from build123d import *

# Parameters (mm, degrees)
SKETCH_1_R          = 3
EXTRUDE_1_DEPTH     = 12
CUT_EXTRUDE_1_DEPTH = 41.249223595
CUT_EXTRUDE_2_DEPTH = 23
SKETCH_4_R          = 2
CUT_EXTRUDE_3_DEPTH = 3
SKETCH_4_2_R        = 2
CUT_EXTRUDE_4_DEPTH = 41.249223625


with BuildPart() as part:
    # Sketch 1 → Extrude 1 (new body)
    with BuildSketch(Plane(origin=(0, 0, 0), x_dir=(1, 0, 0), z_dir=(0, 1, 0))):
        with BuildLine():
            Line((0, 0), (30, 0))
            Line((30, 0), (30, -24))
            Line((30, -24), (10.696938457, -24))
            ThreePointArc((10.696938457, -24), (8.799571861, -23.323790008), (7.757550765, -21.6))
            ThreePointArc((7.757550765, -21.6), (5.601317771, -16.801757364), (1.6, -13.386800671))
            ThreePointArc((1.6, -13.386800671), (0.430953484, -12.282694177), (0, -10.733500839))
            Line((0, -10.733500839), (0, 0))
        make_face()
        with Locations(Location((12, -20, 0), (0, 0, 270))):
            Circle(SKETCH_1_R, mode=Mode.SUBTRACT)
        with Locations(Location((25, -20, 0), (0, 0, 270))):
            Circle(SKETCH_1_R, mode=Mode.SUBTRACT)
    extrude(amount=EXTRUDE_1_DEPTH)

    # Sketch 2 → Cut-Extrude 1 (cut, through all)
    with BuildSketch(Plane(origin=(0, 0, 0), x_dir=(-1, 0, 0), z_dir=(0, 0, -1))):
        with BuildLine():
            Line((-30, 12), (-30, 0))
            ThreePointArc((-30, 0), (-28.649110641, 6), (-30, 12))
        make_face()
    extrude(amount=-CUT_EXTRUDE_1_DEPTH, mode=Mode.SUBTRACT)

    # Sketch 3 → Cut-Extrude 2 (cut)
    with BuildSketch(Plane.ZY):
        Polygon((0, 2.75), (0, 9.25), (4.253461365, 10), (4.253461365, 2), align=None)
    extrude(amount=-CUT_EXTRUDE_2_DEPTH, mode=Mode.SUBTRACT)

    # Sketch 4 → Cut-Extrude 3 (cut)
    with BuildSketch(Plane.ZY):
        with BuildLine():
            Line((4.253461365, 10), (4.253461365, 2))
            ThreePointArc((4.253461365, 2), (11.421253901, 6), (4.253461365, 10))
        make_face()
        with Locations((6.721253901, 6)):
            Circle(SKETCH_4_R, mode=Mode.SUBTRACT)
    extrude(amount=-CUT_EXTRUDE_3_DEPTH, mode=Mode.SUBTRACT)

    # Sketch 4_2 → Cut-Extrude 4 (cut, through all)
    with BuildSketch(Plane.ZY):
        with Locations((6.721253901, 6)):
            Circle(SKETCH_4_2_R)
    extrude(amount=-CUT_EXTRUDE_4_DEPTH, mode=Mode.SUBTRACT)


solid = part.part
Check sheet for the modelled part. Datum: model origin and axes. Units: mm. A direction names the side the tool comes from. Round coordinates to 2 decimals unless told otherwise and drop trailing zeros. Order: outer loops, then holes, each group sorted by start corner. A loop starts at its lowest first (then second) coordinate and runs counter-clockwise, first axis right, second up.
(1) Cross-section at A-A, the plane x = 12. Enter the section's corners in (y, z), and give its area (3 significant figures).
(2) Access from +Z, -Z, +X, -X, +Y, -Y to the whole of each face (thin tool, end or side, straight path). Record for faces 5 (the flat face through (11.34, 9.62, 2.1)), 6 (the cylindrical face through (28.65, 5.91, 11.83)).
(3) Scan lines: probe 1 along X at (y, z) = (5.25, 20); probe 2 along X at (y, z) = (6, 2); probe 3 along X at (y, z) = (8.5, 19.5). Record each from-to range of solid material in increasing order.
(4) Go/stop test with flat-tipped pins: P1, Ø1.5, axis at y = 4, z = 16, coming from the +X side; P2, Ø6.5, axis at x = 9, y = 7, coming from the -Z side; P3, Ø2.5, axis at y = 6, z = 6.72, coming from the -X side; P4, Ø1.3, axis at y = 7, z = 3, coming from the -X side. Record where each tip stops, or that it passes through.
(5) Cross-section at C-C, the plane x = 21. Enter the section's corners in (y, z).
(6) Cross-section at B-B, the plane y = 4.5. Enter the section's corners in (x, z).
(7) Cross-section at D-D, the plane z = 22.5. Enter the section's corners in (x, y), and give its area (3 significant figures).
(8) Draft check along X on faces 1 (the cylindrical face through (12, 6, 17)), 2 (the flat face through (13, 6, 4.253)), 3 (the cylindrical face through (25, 6, 17)), 4 (the cylindrical face through (5.646, 5.916, 16.861)). Enter one of: pulls with the +X half, pulls with the -X half, needs draft (parallel to the pull), parting line crosses it, or undercut.
Check sheet entries:
1. outline: (0, 0) - (2.75, 0) - (2, 4.25) - (10, 4.25) - (9.25, 0) - (12, 0) - (12, 17) - (0, 17) - close; (0, 23) - (12, 23) - (12, 24) - (0, 24) - close; hole circle Ø4 at (6, 6.72)
1. area: 173 mm2
2. face 5: -X
2. face 6: +Z, -Z, +X
3. probe 1: x = 7.31 to 9, 15 to 22, 28 to 28.67
3. probe 2: x = 23 to 28.65
3. probe 3: x = 7.12 to 9.04, 14.96 to 22.04, 27.96 to 28.87
4. P1: stops at x = 28.92
4. P2: stops at z = 0
4. P3: passes through
4. P4: stops at x = 23
5. outline: (0, 0) - (2.75, 0) - (2, 4.25) - (10, 4.25) - (9.25, 0) - (12, 0) - (12, 24) - (0, 24) - close; hole circle Ø4 at (6, 6.72)
6. outline: (0.03, 11.18) - (3, 11.18) - (3, 8.04) - (28.73, 8.04) - (28.73, 24) - (10.7, 24) arc R3 ccw to (7.76, 21.6) arc R12 cw to (1.6, 13.39) arc R3 ccw to start; (3, 4.25) - (23, 4.25) - (23, 0) - (28.73, 0) - (28.73, 5.4) - (3, 5.4) - close; hole circle Ø6 at (12, 20); hole circle Ø6 at (25, 20)
7. outline: (8.1, 0) - (10.34, 0) - (10.34, 12) - (8.1, 12) - close; (13.66, 0) - (23.34, 0) - (23.34, 12) - (13.66, 12) - close; (26.66, 0) - (30, 0) arc R14 cw to (30, 12) - (26.66, 12) - close
7. area: 172 mm2
8. face 1: undercut
8. face 2: needs draft
8. face 3: undercut
8. face 4: pulls with the -X half
